The figure shows three views and two pictorial views of one solid part (mm, origin at its lowest corner). Answer the questions. A direction names the side the tool comes from. Coordinates: 2 decimals unless noted, no trailing zeros. Loops run counter-clockwise (first coordinate to the right, second up) from the corner with the lowest first, then second, coordinate; pieces in that order, holes last. Notation, with made-up numbers: M 72,80.25 L 128,80.25 A23 ccw 128,94.25 Z; hole C 7.5,15 d8. An arc over 180 degrees is marked long. Answer in a Markdown table with one row per item. Add a question column.
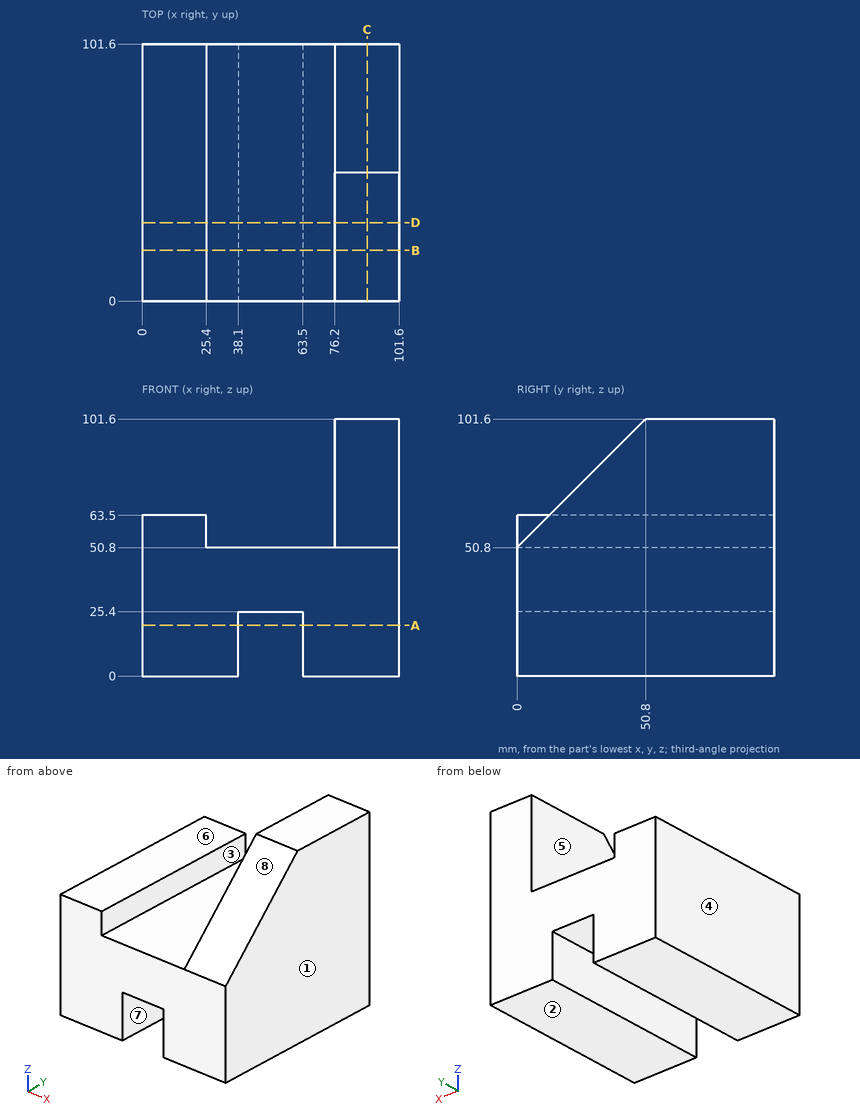
(1) Each of these flat-tipped pins is pushed along its axis until it touches: pin 1 (12.5 mm diameter, centred on x = 9.5, y = 41, fed in from +Z); pin 2 (1 mm diameter, centred on y = 36.5, z = 82, fed in from -X); pin 3 (7.5 mm diameter, centred on x = 50, y = 66, fed in from -Z). Where does it stop, or does it pass through?
(2) A cutting plane is placed at C-C (x = 89). Give the vertices of the cut face in (y, z).
(3) A cutting plane is placed at D-D (y = 31). Give the vertices of the cut face in (x, z).
(4) A cutting plane is placed at B-B (y = 20). Give the vertices of the cut face in (x, z).
(5) The mould has two halves that part along X. Classify the marked faces 1, 2, 3 and 4: released by +X, released by -X, zero draft, split by the parting line, or undercut.
(6) For the marked faces 5, 6, 7 and 8, determine the directions among +Z, -Z, +X, -X, +Y, -Y from which every point of the face is accessible in a straight line to the end or side of a thin tool.
(7) A cutting plane is placed at A-A (z = 20). Give the vertices of the cut face in (x, y).
(8) Straight lines are drawn through the part: line 1 (X direction, y = 61, z = 16.5); line 2 (X direction, y = 24.5, z = 53); line 3 (Z direction, x = 35, y = 73). For each, find the intervals that lie inside material, in ascending order.
Solved:
| question | item | result |
|---|---|---|
| 1 | pin 1 | stops at z = 63.5 |
| 1 | pin 2 | stops at x = 76.2 |
| 1 | pin 3 | stops at z = 25.4 |
| 2 | outline | M 0,0 L 101.6,0 L 101.6,101.6 L 50.8,101.6 L 0,50.8 Z |
| 3 | outline | M 0,0 L 38.1,0 L 38.1,25.4 L 63.5,25.4 L 63.5,0 L 101.6,0 L 101.6,81.8 L 76.2,81.8 L 76.2,50.8 L 25.4,50.8 L 25.4,63.5 L 0,63.5 Z |
| 4 | outline | M 0,0 L 38.1,0 L 38.1,25.4 L 63.5,25.4 L 63.5,0 L 101.6,0 L 101.6,70.8 L 76.2,70.8 L 76.2,50.8 L 25.4,50.8 L 25.4,63.5 L 0,63.5 Z |
| 5 | face 1 | released by +X |
| 5 | face 2 | zero draft |
| 5 | face 3 | undercut |
| 5 | face 4 | released by -X |
| 6 | face 5 | +Z, +Y, -Y |
| 6 | face 6 | +Z, -X, +Y, -Y |
| 6 | face 7 | -Z, +Y, -Y |
| 6 | face 8 | +Z, +X, -Y |
| 7 | outline | M 0,0 L 38.1,0 L 38.1,101.6 L 0,101.6 Z; M 63.5,0 L 101.6,0 L 101.6,101.6 L 63.5,101.6 Z |
| 8 | line 1 | x = 0 to 38.1, 63.5 to 101.6 |
| 8 | line 2 | x = 0 to 25.4, 76.2 to 101.6 |
| 8 | line 3 | z = 0 to 50.8 |
